Model file for the job. Use its own axes, mm. A direction names the side the tool comes from. Coordinates: 2 decimals unless noted, no trailing zeros. Order: outer loops, then holes, each group sorted by start corner. A loop starts at its lowest first (then second) coordinate and runs counter-clockwise, first axis right, second up. Notation, with made-up numbers: (-5, 87) -> (20, 87) arc R14 cw to (20, 113) -> close; hole circle Ø5 at (-36.75, -2). An arc over 180 degrees is marked (long way). Use CSV: the item, a comma, the result in double quotes. Start each with the question number.
(1) Cut at B-B on x = -15. Write the cut outline in (y, z).
(2) Pin check, flat tips, straight feed: pin 1 Ø6 at (y, z) = (-32.5, -5) entering from +X; pin 2 Ø2 at (y, z) = (-1.5, -20.5) entering from +X; pin 3 Ø0.5 at (x, y) = (-1, -16) entering from +Z. Stop position of each tip, or through.
(3) Cut at A-A on y = -22. Write the cut outline in (x, z) (1 decimal).
(4) Probe L1, parallel to Z at x = 6, y = -2; L2, parallel to Z at x = -47.5, y = -33.5; L3, parallel to X at y = -43, z = 7.5. List the from-to ranges inside material, lowest first.
(5) Cut at D-D on z = -15. Write the cut outline in (x, y), plus the area to 3 significant figures.
(6) Cut at C-C on z = -6. Write the cut outline in (x, y), plus the area to 3 significant figures.
(7) Tool access for faces 1 (the flat face through (-0.459, -21, -11)), 2 (the flat face through (8, 0, -32)), 3 (the cylindrical face through (-35.928, -24.65, -31.438)): list every direction of +Z, -Z, +X, -X, +Y, -Y with a clear straight run to the whole face (end or side of a thin tool).
(8) Pull direction Z, two halves, no side cores. Call faces 4 (the flat face through (-2, -50, -1)), 5 (the cylindrical face through (-35.87, -24.65, 29.23)), 6 (the flat face through (-1, -21, -28.609)), 7 (the cylindrical face through (35.05, 3.04, -38.36)): pulls with the +Z half, pulls with the -Z half, needs draft (parallel to the pull), parting line crosses it, or undercut.
```python
from build123d import *

# Parameters (mm, degrees)
BOSS_EXTRUDE1_DEPTH = 6
FILLET1_R           = 20
SKETCH4_W           = 3
SKETCH4_H           = 50
SKETCH6_R           = 16.245672788
CUT_EXTRUDE1_DEPTH  = 10
BOSS_EXTRUDE2_DEPTH = 3
CUT_EXTRUDE2_DEPTH  = 44
BOSS_EXTRUDE3_DEPTH = 53


with BuildPart() as part:
    # Sketch1 → Boss-Extrude1 (new body)
    with BuildSketch(Plane(origin=(0, 0, 0), x_dir=(1, 0, 0), z_dir=(0, 1, 0))):
        with BuildLine():
            Line((34.540516942, 38.609131748), (-36.459483058, 38.609131748))
            ThreePointArc((-36.459483058, 38.609131748), (-66.459483058, 1.109131748), (-36.459483058, -36.390868252))
            Line((-36.459483058, -36.390868252), (34.540516942, -36.390868252))
            ThreePointArc((34.540516942, -36.390868252), (64.540516942, 1.109131748), (34.540516942, 38.609131748))
        make_face()
    extrude(amount=BOSS_EXTRUDE1_DEPTH)

    # Fillet1
    fillet1_edges = [part.edges().sort_by_distance(p)[0] for p in [
        (-36.459483058, 3, -38.609131748),
        (34.540516942, 3, -38.609131748),
        (34.540516942, 3, 36.390868252),
        (-36.459483058, 3, 36.390868252),
    ]]
    fillet(fillet1_edges, radius=FILLET1_R)

    # Sweep1: sweep along a path in Sketch3
    with BuildLine(Plane.XZ) as sweep1_path:
        Line((31.907446823, 29.390868252), (-33.82641294, 29.390868252))
        ThreePointArc((-33.82641294, 29.390868252), (-35.899239553, 29.224550102), (-37.919027907, 28.729851303))
        ThreePointArc((-37.919027907, 28.729851303), (-59.459483058, -1.109131748), (-37.919027907, -30.948114799))
        ThreePointArc((-37.919027907, -30.948114799), (-35.899239553, -31.442813598), (-33.82641294, -31.609131748))
        Line((-33.82641294, -31.609131748), (31.907446823, -31.609131748))
        ThreePointArc((31.907446823, -31.609131748), (33.980273437, -31.442813598), (36.000061791, -30.948114799))
        ThreePointArc((36.000061791, -30.948114799), (57.540516942, -1.109131748), (36.000061791, 28.729851303))
        ThreePointArc((36.000061791, 28.729851303), (33.980273437, 29.224550102), (31.907446823, 29.390868252))
    # Sketch4 → Sweep1 (sweep)
    with BuildSketch(Plane(origin=(31.907446823, 0, -31.609131748), x_dir=(0, 0, -1), z_dir=(1, 0, 0))):
        with Locations((-1.5, -25)):
            Rectangle(SKETCH4_W, SKETCH4_H)
    sweep(path=sweep1_path.line)

    # Sketch6 → Cut-Extrude1 (cut)
    with BuildSketch(Plane(origin=(0, 0, 0), x_dir=(1, 0, 0), z_dir=(0, 1, 0))):
        with Locations((75, 0)):
            Circle(SKETCH6_R)
        with Locations((-76.918966117, 0)):
            Circle(SKETCH6_R)
    extrude(amount=CUT_EXTRUDE1_DEPTH, mode=Mode.SUBTRACT)

    # Sketch7 → Boss-Extrude2 (add)
    with BuildSketch(Plane.XZ.offset(50)):
        with BuildLine():
            Line((31.907446823, 26.390868252), (-33.82641294, 26.390868252))
            ThreePointArc((-33.82641294, 26.390868252), (-35.42089495, 26.262931214), (-36.974578299, 25.882393676))
            ThreePointArc((-36.974578299, 25.882393676), (-56.459483058, -1.109131748), (-36.974578299, -28.100657171))
            ThreePointArc((-36.974578299, -28.100657171), (-35.42089495, -28.481194709), (-33.82641294, -28.609131748))
            Line((-33.82641294, -28.609131748), (31.907446823, -28.609131748))
            ThreePointArc((31.907446823, -28.609131748), (33.501928834, -28.481194709), (35.055612183, -28.100657171))
            ThreePointArc((35.055612183, -28.100657171), (54.540516942, -1.109131748), (35.055612183, 25.882393676))
            ThreePointArc((35.055612183, 25.882393676), (33.501928834, 26.262931214), (31.907446823, 26.390868252))
        make_face()
    extrude(amount=-BOSS_EXTRUDE2_DEPTH)

    # Sketch9 → Cut-Extrude2 (cut)
    with BuildSketch(Plane.XZ):
        with BuildLine():
            Line((-33.82641294, -28.609131748), (31.907446823, -28.609131748))
            ThreePointArc((31.907446823, -28.609131748), (33.501928834, -28.481194709), (35.055612183, -28.100657171))
            ThreePointArc((35.055612183, -28.100657171), (54.540516942, -1.109131748), (35.055612183, 25.882393676))
            ThreePointArc((35.055612183, 25.882393676), (33.501928834, 26.262931214), (31.907446823, 26.390868252))
            Line((31.907446823, 26.390868252), (-33.82641294, 26.390868252))
            ThreePointArc((-33.82641294, 26.390868252), (-35.42089495, 26.262931214), (-36.974578299, 25.882393676))
            ThreePointArc((-36.974578299, 25.882393676), (-56.459483058, -1.109131748), (-36.974578299, -28.100657171))
            ThreePointArc((-36.974578299, -28.100657171), (-35.42089495, -28.481194709), (-33.82641294, -28.609131748))
        make_face()
    extrude(amount=-CUT_EXTRUDE2_DEPTH, mode=Mode.SUBTRACT)

    # Sketch10 → Boss-Extrude3 (add)
    with BuildSketch(Plane(origin=(0, -47, 0), x_dir=(1, 0, 0), z_dir=(0, 1, 0))):
        Polygon((-0.459483058, 1.609131748), (44.905858694, 1.609131748), (44.905858694, 0.609131748), (-0.459483058, 0.609131748), (-0.459483058, -22.435523008), (-1.459483058, -22.435523008), (-1.459483058, 0.609131748), (-49.663240978, 0.609131748), (-49.663240978, 1.609131748), (-1.459483058, 1.609131748), (-1.459483058, 20.900521065), (-0.459483058, 20.900521065), align=None)
    extrude(amount=BOSS_EXTRUDE3_DEPTH)


solid = part.part
```
Outcome:
1,outline,"(-50, -31.61) -> (0, -31.61) -> (0, -38.61) -> (6, -38.61) -> (6, -28.61) -> (-47, -28.61) -> (-47, -1.61) -> (6, -1.61) -> (6, -0.61) -> (-47, -0.61) -> (-47, 26.39) -> (6, 26.39) -> (6, 36.39) -> (0, 36.39) -> (0, 29.39) -> (-50, 29.39) -> close"
2,pin 1,"x = 57.53"
2,pin 2,"x = 51.6"
2,pin 3,"z = 29.39"
3,outline,"(-49.7, -1.6) -> (-1.5, -1.6) -> (-1.5, -20.9) -> (-0.5, -20.9) -> (-0.5, -1.6) -> (44.9, -1.6) -> (44.9, -0.6) -> (-0.5, -0.6) -> (-0.5, 22.4) -> (-1.5, 22.4) -> (-1.5, -0.6) -> (-49.7, -0.6) -> close; (-37.9, -30.9) arc R13 ccw to (-33.8, -31.6) -> (31.9, -31.6) arc R13 ccw to (36, -30.9) arc R31.4 ccw to (36, 28.7) arc R13 ccw to (31.9, 29.4) -> (-33.8, 29.4) arc R13 ccw to (-37.9, 28.7) arc R31.4 ccw to start; hole (-37, -28.1) arc R10 ccw to (-33.8, -28.6) -> (31.9, -28.6) arc R10 ccw to (35.1, -28.1) arc R28.4 ccw to (35.1, 25.9) arc R10 ccw to (31.9, 26.4) -> (-33.8, 26.4) arc R10 ccw to (-37, 25.9) arc R28.4 ccw to start"
4,L1,"-31.61 to -28.61, -1.61 to -0.61, 26.39 to 29.39"
4,L2,"-25.79 to -21.83, -1.61 to -0.61, 19.61 to 23.57"
4,L3,"-58.26 to -55.13, -1.46 to -0.46, 53.21 to 56.34"
5,outline,"(-63.86, 0) -> (-56.22, 0) -> (-56.22, -50) -> (54.31, -50) -> (54.31, 0) -> (61.94, 0) -> (61.94, 6) -> (50.92, 6) -> (50.92, -47) -> (-0.46, -47) -> (-0.46, 6) -> (-1.46, 6) -> (-1.46, -47) -> (-52.84, -47) -> (-52.84, 6) -> (-63.86, 6) -> close"
5,area,"835 mm2"
6,outline,"(-61.82, 0) -> (-59.08, 0) -> (-59.08, -50) -> (57.16, -50) -> (57.16, 0) -> (59.9, 0) -> (59.9, 6) -> (54.12, 6) -> (54.12, -47) -> (-0.46, -47) -> (-0.46, 6) -> (-1.46, 6) -> (-1.46, -47) -> (-56.04, -47) -> (-56.04, 6) -> (-61.82, 6) -> close"
6,area,"757 mm2"
7,face 1,"+Y"
7,face 2,"-Y"
7,face 3,"-Z, -X, -Y"
8,face 4,"needs draft"
8,face 5,"pulls with the +Z half"
8,face 6,"undercut"
8,face 7,"pulls with the -Z half"
